Geometry check sheet. Reference: the model listing, model coordinates, mm. A direction names the side the tool comes from. Round coordinates to 2 decimals unless told otherwise and drop trailing zeros. Loops run counter-clockwise (first coordinate to the right, second up) from the corner with the lowest first, then second, coordinate; pieces in that order, holes last. Notation, with made-up numbers: (6.25, -21) - (17.25, -21) arc R11 ccw to (17.25, -17) - close; hole circle Ø6 at (13.25, -26). An arc over 180 degrees is marked (long way). Answer as CSV lines item,"result". Start each with the question number.
1) Cross-section at B-B on z = 20. Record the boundary of the cut face in (x, y), and give its area (3 significant figures).
2) Cross-section at A-A on x = 45. Record the boundary of the cut face in (y, z).
3) Thickness scan on line 1 along Z through (x, y) = (45, -12.5); line 2 along X through (y, z) = (-16.25, 31); line 3 along Z through (x, y) = (6.5, -17). Record the ranges inside material, lowest first.
4) Cross-section at C-C on y = -4.75. Record the boundary of the cut face in (x, z), and give its area (3 significant figures).
5) Cross-section at D-D on x = -13.5. Record the boundary of the cut face in (y, z).
6) Draft check along Z on faces 3 (the cylindrical face through (53, -12, 20)), 4 (the flat face through (45, -12, 40)), 5 (the flat face through (-1, 0, -3)). Enter one of: released by +Z, released by -Z, zero draft, split by the parting line, or undercut.
7) Access from +Z, -Z, +X, -X, +Y, -Y to the whole of each face (thin tool, end or side, straight path). Record for faces 1 (the flat face through (-45, -12, 40)), 2 (the flat face through (-30, -13, 19)).
8) Depth check by flat-ended pin: P1, Ø9.5, axis at x = -45, z = 20, coming from the +Y side; P2, Ø7.5, axis at x = -12.5, y = -15, coming from the +Z side. Enter the tip coordinate at first touch or a pass-through.
from build123d import *

# Parameters (mm, degrees)
F0_W      = 60
F0_H      = 40
F0_R      = 8
F1_DEPTH  = 25
F2_FACE_W = 120
F2_FACE_H = 25
F3_DEPTH  = 20
F4_W      = 60
F4_H      = 42
F5_DEPTH  = 25.001


with BuildPart() as f1:
    # F0 (on Front) → F1 (new body)
    with BuildSketch(Plane.XZ):
        with Locations((-30, 20)):
            Rectangle(F0_W, F0_H)
        with Locations((-45, 20)):
            Circle(F0_R, mode=Mode.SUBTRACT)
    extrude(amount=F1_DEPTH)

    # F2: F1 across face


with BuildPart() as f1_1:
    add(f1.part)
    add(f1.part.mirror(Plane(origin=(0, -12.5, 20), x_dir=(0, 1, 0), z_dir=(1, 0, 0))))

    # F2_face (on face) → F3 (join)
    with BuildSketch(Plane(origin=(0, -12.5, 0), x_dir=(1, 0, 0), z_dir=(0, 0, -1))):
        Rectangle(F2_FACE_W, F2_FACE_H)
    extrude(amount=F3_DEPTH)

    # F4 (on face) → F5 (cut, through all)
    with BuildSketch(Plane.XZ.offset(25)):
        with Locations((0, 19)):
            Rectangle(F4_W, F4_H)
    extrude(amount=-F5_DEPTH, mode=Mode.SUBTRACT)


solid = f1_1.part
Answer block:
1,outline,"(-60, -25) - (-53, -25) - (-53, 0) - (-60, 0) - close; (-37, -25) - (-30, -25) - (-30, 0) - (-37, 0) - close; (30, -25) - (37, -25) - (37, 0) - (30, 0) - close; (53, -25) - (60, -25) - (60, 0) - (53, 0) - close"
1,area,"700 mm^2"
2,outline,"(-25, -20) - (0, -20) - (0, 12) - (-25, 12) - close; (-25, 28) - (0, 28) - (0, 40) - (-25, 40) - close"
3,line 1,"z = -20 to 12, 28 to 40"
3,line 2,"x = -60 to -30, 30 to 60"
3,line 3,"z = -20 to -2"
4,outline,"(-60, -20) - (60, -20) - (60, 40) - (30, 40) - (30, -2) - (-30, -2) - (-30, 40) - (-60, 40) - close; hole circle Ø16 at (-45, 20); hole circle Ø16 at (45, 20)"
4,area,"4,280 mm^2"
5,outline,"(-25, -20) - (0, -20) - (0, -2) - (-25, -2) - close"
6,face 3,"undercut"
6,face 4,"released by +Z"
6,face 5,"zero draft"
7,face 1,"+Z, +X, -X, +Y, -Y"
7,face 2,"+Z, +Y, -Y"
8,P1,"passes through"
8,P2,"stops at z = -2"
